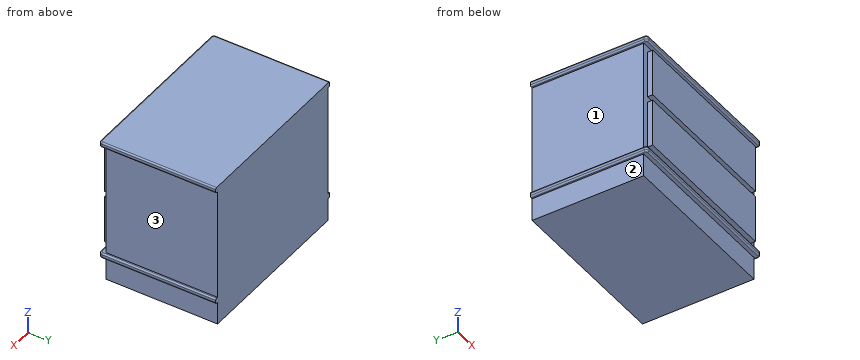
```python
from build123d import *

# Parameters (mm, degrees)
F0_W      = 605
F0_H      = 405
F1_DEPTH  = 505
F2_W      = 10
F2_H      = 389
F2_H_2    = 80
F3_DEPTH  = 410
F4_W      = 18
F4_H      = 389
F4_H_2    = 80
F5_DEPTH  = 610
F7_DEPTH  = 510
F8_R      = 5
F9_W      = 545
F9_H      = 164
F9_H_2    = 165
F10_DEPTH = 18


with BuildPart() as f1:
    # F0 (on Top) → F1 (new body)
    with BuildSketch(Plane.XY):
        with Locations((-302.5, 202.5)):
            Rectangle(F0_W, F0_H)
    extrude(amount=F1_DEPTH)

    # F2 (on face) → F3 (cut)
    with BuildSketch(Plane.XZ):
        with Locations((-600, 292.5)):
            Rectangle(F2_W, F2_H)
        with Locations((-600, 40)):
            Rectangle(F2_W, F2_H_2)
        with Locations((-5, 292.5)):
            Rectangle(F2_W, F2_H)
        with Locations((-5, 40)):
            Rectangle(F2_W, F2_H_2)
    extrude(amount=-F3_DEPTH, mode=Mode.SUBTRACT)

    # F4 (on face) → F5 (cut)
    with BuildSketch(Plane(origin=(-595, 0, 0), x_dir=(0, -1, 0), z_dir=(-1, 0, 0))):
        with Locations((-9, 292.5)):
            Rectangle(F4_W, F4_H)
        with Locations((-9, 40)):
            Rectangle(F4_W, F4_H_2)
    extrude(amount=-F5_DEPTH, mode=Mode.SUBTRACT)

    # F6 (on face) → F7 (cut)
    with BuildSketch(Plane.XY.offset(505)):
        with BuildLine():
            ThreePointArc((-595, 0), (-602.0710678119, 2.9289321881), (-605, 10))
            Line((-605, 10), (-605, 0))
            Line((-605, 0), (-595, 0))
        make_face()
        with BuildLine():
            Line((0, 0), (0, 10))
            ThreePointArc((0, 10), (-2.9289321881, 2.9289321881), (-10, 0))
            Line((-10, 0), (0, 0))
        make_face()
    extrude(amount=-F7_DEPTH, mode=Mode.SUBTRACT)

    # F8
    f8_edges = [f1.edges().sort_by_distance(p)[0] for p in [
        (-302.5, 0, 505),
        (-302.5, 0, 487),
        (-302.5, 0, 98),
        (-302.5, 0, 80),
    ]]
    fillet(f8_edges, radius=F8_R)

    # F9 (on face) → F10 (join)
    with BuildSketch(Plane.XZ.offset(-18)):
        with Locations((-302.5, 385)):
            Rectangle(F9_W, F9_H)
        with Locations((-302.5, 200.5)):
            Rectangle(F9_W, F9_H_2)
    extrude(amount=F10_DEPTH)


solid = f1.part
```
The model under review builds one solid part; all positions refer to its coordinate system, in mm. Face numbers are marked on the shaded views. A direction names the side the tool comes from. Give positions to 0.01 mm unless a question says otherwise; leave off trailing zeros. Write each loop counter-clockwise with the first axis right and the second up, starting at its lowest first coordinate (ties: lowest second). Pieces come first, ordered by that corner, then holes. Notation, with made-up numbers: (22.25, 14) -> (45.25, 14) arc R9 cw to (45.25, 31) -> close; hole circle Ø7 at (-38.75, 64). An arc over 180 degrees is marked (long way). Answer in a Markdown table with one row per item.
1) Add section B-B on y = 72. State the section outline as (x, z) points.
Worked answers:
| item | result |
|---|---|
| outline | (-605, 85) arc R5 ccw to (-600, 80) -> (-595, 80) -> (-595, 0) -> (-10, 0) -> (-10, 80) -> (-5, 80) arc R5 ccw to (0, 85) -> (0, 93) arc R5 ccw to (-5, 98) -> (-10, 98) -> (-10, 487) -> (-5, 487) arc R5 ccw to (0, 492) -> (0, 500) arc R5 ccw to (-5, 505) -> (-600, 505) arc R5 ccw to (-605, 500) -> (-605, 492) arc R5 ccw to (-600, 487) -> (-595, 487) -> (-595, 98) -> (-600, 98) arc R5 ccw to (-605, 93) -> close |
2) Tool access review of the marked faces 1, 2 and 3: name each direction out of +Z, -Z, +X, -X, +Y, -Y from which nothing blocks a thin tool from reaching the whole face with its end or side.
Worked answers:
| item | result |
|---|---|
| face 1 | -X, +Y, -Y |
| face 2 | -Z, -X, +Y, -Y |
| face 3 | +X, +Y, -Y |
3) Add section A-A on z = 182.5. State the section outline as (x, y) points, plus the area to 3 significant figures.
Worked answers:
| item | result |
|---|---|
| outline | (-595, 18) -> (-575, 18) -> (-575, 0) -> (-30, 0) -> (-30, 18) -> (-10, 18) -> (-10, 405) -> (-595, 405) -> close |
| area | 236,000 mm² |
4) Clearance check with flat-ended pins moving along their axes: P1, Ø5.5, axis at y = 7, z = 224, coming from the +X side; P2, Ø14.5, axis at y = 12, z = 352, coming from the +X side; P3, Ø10, axis at y = 324.5, z = 216.5, coming from the -X side. State where each tip first meets the part, or that it passes through.
Worked answers:
| item | result |
|---|---|
| P1 | x = -30 |
| P2 | x = -10 |
| P3 | x = -595 |
5) For L1, parallel to Y at x = -48, z = 111; L2, parallel to X at y = 335, z = 438.5, list the stretches that pass through material, from the lowest coordinate up. Write a range as [from, to].
Worked answers:
| item | result |
|---|---|
| L1 | [18, 405] |
| L2 | [-595, -10] |
